The drawing under review shows one solid part. Ordinate dimensions are in mm from its lowest x, y, z. A direction names the side the tool comes from. Round coordinates to 2 decimals unless told otherwise and drop trailing zeros. Loops run counter-clockwise (first coordinate to the right, second up) from the corner with the lowest first, then second, coordinate; pieces in that order, holes last. Notation, with made-up numbers: M -35,2.25 L -14,2.25 A21 cw -14,22.25 Z; hole C 88,-38.75 d1. An arc over 180 degrees is marked long. Use a Markdown table: item, result.
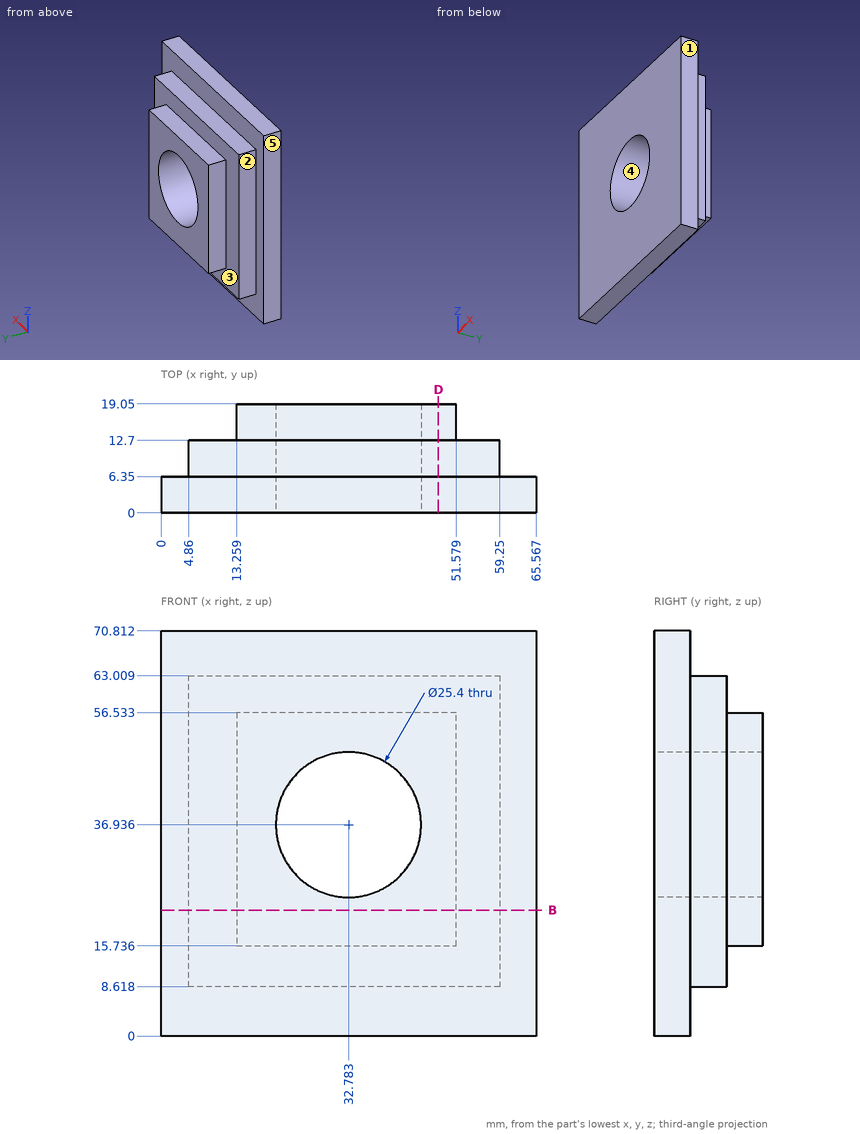
1. Take a section at D-D on x = 48.5. Give the boundary of the cut face in (y, z), and give its area (3 significant figures).
Check values:
| item | result |
|---|---|
| outline | M 0,0 L 6.35,0 L 6.35,8.62 L 12.7,8.62 L 12.7,15.74 L 19.05,15.74 L 19.05,56.53 L 12.7,56.53 L 12.7,63.01 L 6.35,63.01 L 6.35,70.81 L 0,70.81 Z |
| area | 1,050 mm² |
2. Machinability: for the marked faces 1 and 2, which of the approach directions +Z, -Z, +X, -X, +Y, -Y give a long, thin tool a straight path to every point of the face, cutting with its end or side? Answer none if there is none.
Check values:
| item | result |
|---|---|
| face 1 | +Z, -Z, +X, +Y, -Y |
| face 2 | +Z, -Z, -X, +Y |
3. Insertion check: pin 1 (5 mm diameter, centred on y = 9.5, z = 44, fed in from +X); pin 2 (1.9 mm diameter, centred on x = 38.5, y = 9, fed in from -Z); pin 3 (6 mm diameter, centred on y = 7, z = 35.5, fed in from +X); pin 4 (15 mm diameter, centred on x = 32.78, z = 36.94, fed in from +Y). Each pin has a flat end and moves straight along its axis. Give the tip position at first contact, or say it passes through.
Check values:
| item | result |
|---|---|
| pin 1 | stops at x = 59.25 |
| pin 2 | stops at z = 8.62 |
| pin 3 | stops at x = 65.57 |
| pin 4 | passes through |
4. Take a section at B-B on z = 22. Give the boundary of the cut face in (x, y).
Check values:
| item | result |
|---|---|
| outline | M 0,0 L 65.57,0 L 65.57,6.35 L 59.25,6.35 L 59.25,12.7 L 51.58,12.7 L 51.58,19.05 L 13.26,19.05 L 13.26,12.7 L 4.86,12.7 L 4.86,6.35 L 0,6.35 Z |
5. Wall thickness on line 1 along X through (y, z) = (6.5, 37.5); line 2 along X through (y, z) = (2, 37); line 3 along Y through (x, z) = (15, 67): over which ranges is each line inside the solid? List them lowest first. Write a range as from..to.
Check values:
| item | result |
|---|---|
| line 1 | x = 4.86..20.1, 45.47..59.25 |
| line 2 | x = 0..20.08, 45.48..65.57 |
| line 3 | y = 0..6.35 |
6. The part is to be moulded in two halves that separate along X. For the marked faces 3, 4 and 5, say which applies: pulls with the +X half, pulls with the -X half, needs draft (parallel to the pull), parting line crosses it, or undercut.
Check values:
| item | result |
|---|---|
| face 3 | needs draft |
| face 4 | undercut |
| face 5 | pulls with the -X half |
